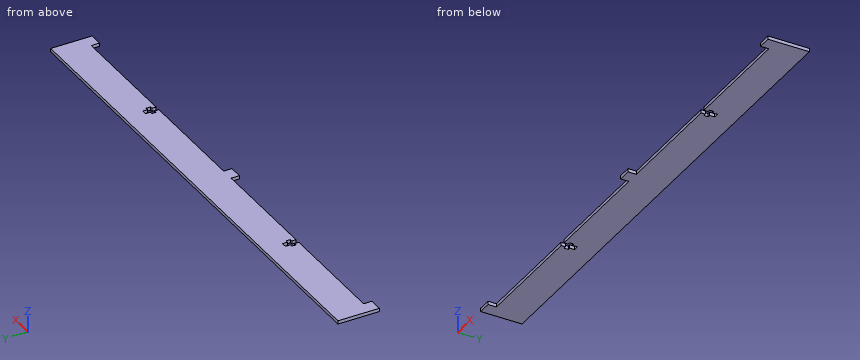
from build123d import *

# Parameters (mm, degrees)
EXTRUDE_1_DEPTH = 2


with BuildPart() as part:
    # 草图1 → 凸台-拉伸1 (new body)
    with BuildSketch(Plane.XY):
        Polygon((-229, 0), (-229, -5), (-221, -5), (-221, 0), (-151.5, 0), (-151.5, 2.5), (-153, 2.5), (-153, 5.1), (-151.5, 5.1), (-151.5, 8.1), (-148.5, 8.1), (-148.5, 5.1), (-147, 5.1), (-147, 2.5), (-148.5, 2.5), (-148.5, 0), (-79, 0), (-79, -5), (-71, -5), (-71, 0), (-1.5, 0), (-1.5, 2.5), (-3, 2.5), (-3, 5.1), (-1.5, 5.1), (-1.5, 8.1), (1.5, 8.1), (1.5, 5.1), (3, 5.1), (3, 2.5), (1.5, 2.5), (1.5, 0), (71, 0), (71, -5), (79, -5), (79, 0), (79, 20), (71, 20), (-229, 20), align=None)
    extrude(amount=EXTRUDE_1_DEPTH)


solid = part.part
Design review of the part built by this model. Coordinates are the model's own, in mm. Coordinates: 2 decimals unless noted, no trailing zeros. Loops run counter-clockwise (first coordinate to the right, second up) from the corner with the lowest first, then second, coordinate; pieces in that order, holes last. Notation, with made-up numbers: M 21,52 L 34,52 A17 cw 34,74 Z; hole C 44,40 d2. An arc over 180 degrees is marked long. Use one line per item in the form item = value.
(1) For line 1 along X through (y, z) = (0.5, 1.3); line 2 along X through (y, z) = (-0.75, 1.35); line 3 along Y through (x, z) = (-20, 1.6), list the stretches that pass through material, from the lowest coordinate up. Write a range as from..to.
Return value:
line_1 = -229..-151.5, -148.5..-1.5, 1.5..79
line_2 = -229..-221, -79..-71, 71..79
line_3 = 0..20
(2) Consider section A-A (x = 14.5). Write out the cut boundary in (y, z).
Return value:
outline = M 0,0 L 20,0 L 20,2 L 0,2 Z
(3) Clearance check with a flat-ended pin moving along its axis: P1, Ø1, axis at x = 51.5, z = 1, coming from the -Y side. State where the tip first meets the part, or that it passes through.
Return value:
P1 = 0
